Build history of the part. All positions in model axes, mm. A direction names the side the tool comes from. Round coordinates to 2 decimals unless told otherwise and drop trailing zeros. Loops run counter-clockwise (first coordinate to the right, second up) from the corner with the lowest first, then second, coordinate; pieces in that order, holes last.
from build123d import *

# Parameters (mm, degrees)
SKETCH1_W           = 10
SKETCH1_H           = 23
SKETCH1_R           = 2.8
BOSS_EXTRUDE1_DEPTH = 6
SKETCH2_W           = 10
SKETCH2_H           = 5
BOSS_EXTRUDE2_DEPTH = 20
SKETCH4_R           = 2.25
CUT_EXTRUDE1_DEPTH  = 10
FILLET1_R           = 2


with BuildPart() as part:
    # Sketch1 → Boss-Extrude1 (new body)
    with BuildSketch(Plane(origin=(0, 0, 0), x_dir=(1, 0, 0), z_dir=(0, 1, 0))):
        with Locations((0, 3.5)):
            Rectangle(SKETCH1_W, SKETCH1_H)
        with Locations(Location((0, 0, 0), (0, 0, 270))):
            Circle(SKETCH1_R, mode=Mode.SUBTRACT)
    extrude(amount=BOSS_EXTRUDE1_DEPTH)

    # Sketch2 → Boss-Extrude2 (add)
    with BuildSketch(Plane(origin=(0, 6, 0), x_dir=(1, 0, 0), z_dir=(0, 1, 0))):
        with Locations((0, 12.5)):
            Rectangle(SKETCH2_W, SKETCH2_H)
    extrude(amount=BOSS_EXTRUDE2_DEPTH)

    # Sketch4 → Cut-Extrude1 (cut)
    with BuildSketch(Plane.XY.offset(-10)):
        with Locations((-1.3, 11.3)):
            Circle(SKETCH4_R)
        with Locations((-1.3, 21.3)):
            Circle(SKETCH4_R)
    extrude(amount=-CUT_EXTRUDE1_DEPTH, mode=Mode.SUBTRACT)

    # Fillet1
    fillet1_edges = [part.edges().sort_by_distance(p)[0] for p in [
        (0, 6, -10),
    ]]
    fillet(fillet1_edges, radius=FILLET1_R)


solid = part.part
(1) Slice it at C-C on x = 4. List the corners of the cut face in (y, z).
Responses:
outline: (0, -15) - (26, -15) - (26, -10) - (8, -10) arc R2 cw to (6, -8) - (6, 8) - (0, 8) - close
(2) Pull direction X, two halves, no side cores. Call faces 1 (the face through (-5, 7, -11)), 2 (the face through (5, 7, -11)), 3 (the face through (-0.09, 13.197, -12.465)), 4 (the face through (1, 13, -15)): +X half, -X half, draft (parallel to the pull), parting line (faces both ways), or undercut.
Responses:
face 1: -X half
face 2: +X half
face 3: undercut
face 4: draft
(3) Which spindle directions (+Z, -Z, +X, -X, +Y, -Y) get a long thin tool onto all of the face, cutting with end or side? Do faces 5 (the face through (-2.3, 6, -1.9)), 6 (the face through (0, 0, -4)). Say none if no direction does.
Responses:
face 5: +Z, +X, -X, +Y
face 6: +Z, -Z, +X, -X, -Y
(4) Slice it at B-B on z = 0. List the corners of the cut face in (x, y).
Responses:
outline: (-5, 0) - (-2.8, 0) - (-2.8, 6) - (-5, 6) - close; (2.8, 0) - (5, 0) - (5, 6) - (2.8, 6) - close
(5) Probe line 1 (Y direction, x = -1.3, z = -13.5); line 2 (X direction, y = 4.6, z = 0); line 3 (Y direction, x = -2, z = -13). List the from-to ranges inside material, lowest first.
Responses:
line 1: y = 0 to 9.05, 13.55 to 19.05, 23.55 to 26
line 2: x = -5 to -2.8, 2.8 to 5
line 3: y = 0 to 9.16, 13.44 to 19.16, 23.44 to 26
(6) Slice it at D-D on z = -13.25. List the corners of the cut face in (x, y).
Responses:
outline: (-5, 0) - (5, 0) - (5, 26) - (-5, 26) - close; hole circle Ø4.5 at (-1.3, 11.3); hole circle Ø4.5 at (-1.3, 21.3)
(7) Pin check, flat tips, straight feed: P1, Ø3.5, axis at x = -1.3, y = 21.3, coming from the -Z side (1 decimal); P2, Ø1, axis at x = -3, y = 12, coming from the +Z side; P3, Ø6, axis at x = -3, z = 0, coming from the +Y side. Stop position of each tip, or through.
Responses:
P1: passes through
P2: stops at z = -10
P3: stops at y = 6
(8) Slice it at A-A on y = 21.3. List the corners of the cut face in (x, z), plus the area to 3 significant figures.
Responses:
outline: (-5, -15) - (-3.55, -15) - (-3.55, -10) - (-5, -10) - close; (0.95, -15) - (5, -15) - (5, -10) - (0.95, -10) - close
area: 27.5 mm2
